from build123d import *

# Parameters (mm, degrees)
SKETCH1_R           = 5
BOSS_EXTRUDE1_DEPTH = 8
SKETCH4_R           = 16
BOSS_EXTRUDE3_DEPTH = 12
SKETCH5_R           = 11
CUT_EXTRUDE3_DEPTH  = 116.108644332


with BuildPart() as part:
    # Sketch1 → Boss-Extrude1 (new body)
    with BuildSketch(Plane.XY):
        with BuildLine():
            Line((-9.871170143, 76.6), (-21.716574315, 3.52))
            ThreePointArc((-21.716574315, 3.52), (-15.360764468, -15.749505229), (4.061538462, -21.62183862))
            Line((4.061538462, -21.62183862), (66.846153846, -9.828108464))
            ThreePointArc((66.846153846, -9.828108464), (74.999999999, -0.000112634), (66.846375241, 9.828066874))
            Line((66.846375241, 9.828066874), (26.145857586, 17.474375048))
            ThreePointArc((26.145857586, 17.474375048), (20.833288171, 20.320356887), (18.121062683, 25.702441922))
            Line((18.121062683, 25.702441922), (9.871170143, 76.6))
            ThreePointArc((9.871170143, 76.6), (0, 85), (-9.871170143, 76.6))
        make_face()
        with Locations((0, 75)):
            Circle(SKETCH1_R, mode=Mode.SUBTRACT)
        with Locations((65, 0)):
            Circle(SKETCH1_R, mode=Mode.SUBTRACT)
    extrude(amount=BOSS_EXTRUDE1_DEPTH)

    # Sketch4 → Boss-Extrude3 (add)
    with BuildSketch(Plane.XY.offset(8)):
        Circle(SKETCH4_R)
    extrude(amount=BOSS_EXTRUDE3_DEPTH)

    # Sketch5 → Cut-Extrude3 (cut, through all)
    with BuildSketch(Plane.XY.offset(20)):
        Circle(SKETCH5_R)
    extrude(amount=-CUT_EXTRUDE3_DEPTH, mode=Mode.SUBTRACT)


solid = part.part
The listing builds one solid part. Answer for the finished solid, in the listing's coordinates (mm). A direction names the side the tool comes from. Give positions to 0.01 mm unless a question says otherwise; leave off trailing zeros. Write each loop counter-clockwise with the first axis right and the second up, starting at its lowest first coordinate (ties: lowest second). Pieces come first, ordered by that corner, then holes.
1) Section D-D (y = 75) is taken. Write down the section's boundary in (x, z), and give its area (3 significant figures).
2) Section A-A (x = 0) is taken. Write down the section's boundary in (y, z), and give its area (3 significant figures).
3) A tool of negligible diameter and unlimited length cuts with its end or side. For faces 5 (the face through (-15.71, 40.57, 3.94)), 6 (the face through (-3.47, -15.62, 13.92)), from which of +Z, -Z, +X, -X, +Y, -Y can it reach the whole face along a straight path? Write none if from no direction.
4) Find the intervals of material crossed by L1, parallel to Y at x = 0, z = 10; L2, parallel to Z at x = -10, y = -14; L3, parallel to Y at x = 65, z = 3.5, in increasing order.
5) Given P1, Ø3, axis at y = 4, z = 11, coming from the -X side; P2, Ø10, axis at y = 33, z = 4, coming from the -X side; P3, Ø6, axis at x = 16, z = 14, coming from the +Y side, each flat-ended and moving along its own axis, determine where each tip first touches the part or whether it passes through.
6) Section C-C (z = 4) is taken. Write down the section's boundary in (x, y).
7) Section B-B (y = 0) is taken. Write down the section's boundary in (x, z).
8) For a pull along Y with two mould halves and no side action, classify faces 1 (the face through (-1.08, 70.12, 3.94)), 2 (the face through (-2.38, -10.74, 10.14)), 3 (the face through (46.781, 13.598, 3.944)), 4 (the face through (75, 0, 4)) as pulls with the +Y half, pulls with the -Y half, needs draft (parallel to the pull), parting line crosses it, or undercut.
Response:
1. outline: (-10.13, 0) - (-5, 0) - (-5, 8) - (-10.13, 8) - close; (5, 0) - (10.13, 0) - (10.13, 8) - (5, 8) - close
1. area: 82.1 mm2
2. outline: (-22, 0) - (-11, 0) - (-11, 20) - (-16, 20) - (-16, 8) - (-22, 8) - close; (11, 0) - (70, 0) - (70, 8) - (16, 8) - (16, 20) - (11, 20) - close; (80, 0) - (85, 0) - (85, 8) - (80, 8) - close
2. area: 720 mm2
3. face 5: +Z, -Z, -X, +Y
3. face 6: +Z
4. L1: y = -16 to -11, 11 to 16
4. L2: z = 0 to 8
4. L3: y = -10.17 to -5, 5 to 10.17
5. P1: stops at x = -15.8
5. P2: stops at x = -17.75
5. P3: stops at y = 9.33
6. outline: (-21.72, 3.52) arc R22 ccw to (4.06, -21.62) - (66.85, -9.83) arc R10 ccw to (66.85, 9.83) - (26.15, 17.47) arc R10 cw to (18.12, 25.7) - (9.87, 76.6) arc R10 ccw to (-9.87, 76.6) - close; hole circle Ø22 at (0, 0); hole circle Ø10 at (0, 75); hole circle Ø10 at (65, 0)
7. outline: (-22, 0) - (-11, 0) - (-11, 20) - (-16, 20) - (-16, 8) - (-22, 8) - close; (11, 0) - (60, 0) - (60, 8) - (16, 8) - (16, 20) - (11, 20) - close; (70, 0) - (75, 0) - (75, 8) - (70, 8) - close
8. face 1: undercut
8. face 2: undercut
8. face 3: pulls with the +Y half
8. face 4: parting line crosses it
